Build history of the part. All positions in model axes, mm. A direction names the side the tool comes from. Give positions to 0.01 mm unless a question says otherwise; leave off trailing zeros. Loops run counter-clockwise (first coordinate to the right, second up) from the corner with the lowest first, then second, coordinate; pieces in that order, holes last. Notation, with made-up numbers: (-20.5, 85) -> (7.5, 85) arc R26 cw to (7.5, 112) -> close; hole circle Ø4 at (51, 73). An arc over 180 degrees is marked (long way). One line per question, with ' | ' between items. Start each with the question number.
(1) Flat gauge pin, fed straight in: pin 1 Ø3 at (x, y) = (50, 15.5) entering from -Z. Where does the tip first touch, or does it go through?
(2) Slice it at A-A, the plane x = 50. Write the cut outline in (y, z).
(3) Drill centre lines: L1, parallel to X at y = 15, z = 8.25; L2, parallel to Y at x = 50, z = 91. Where is each one in solid material? Low to high. Write a range as from..to.
(4) 3-axis set-ups, long thin cutter, end or side, ignore diameter. For faces 4 (the face through (47.6, 16.8, 5.9)), 5 (the face through (49, 0, 49)), 6 (the face through (50, 15, 88)): which of +Z, -Z, +X, -X, +Y, -Y reach the whole face in a straight line?
(5) Mould opens along X. For faces 1 (the face through (50, 15, 12)), 2 (the face through (49, 30, 49)), 3 (the face through (100, 15, 49)) say: pulls with the +X half, pulls with the -X half, needs draft (parallel to the pull), parting line crosses it, or undercut.
```python
from build123d import *

# Parameters (mm, degrees)
F0_W     = 100
F0_H     = 30
F1_DEPTH = 100
F2_R     = 3
F3_DEPTH = 12
F4_R     = 3
F5_DEPTH = 12


with BuildPart() as f1:
    # F0 (on Top) → F1 (new body)
    with BuildSketch(Plane.XY):
        with Locations((50, 15)):
            Rectangle(F0_W, F0_H)
    extrude(amount=F1_DEPTH)

    # F2 (on face) → F3 (cut)
    with BuildSketch(Plane(origin=(0, 0, 0), x_dir=(1, 0, 0), z_dir=(0, 0, -1))):
        with Locations((50, -15)):
            Circle(F2_R)
    extrude(amount=-F3_DEPTH, mode=Mode.SUBTRACT)

    # F4 (on face) → F5 (cut)
    with BuildSketch(Plane.XY.offset(100)):
        with Locations((50, 15)):
            Circle(F4_R)
    extrude(amount=-F5_DEPTH, mode=Mode.SUBTRACT)


solid = f1.part
```
Final values:
1) pin 1: z = 12
2) outline: (0, 0) -> (12, 0) -> (12, 12) -> (18, 12) -> (18, 0) -> (30, 0) -> (30, 100) -> (18, 100) -> (18, 88) -> (12, 88) -> (12, 100) -> (0, 100) -> close
3) L1: 0..47, 53..100 | L2: 0..12, 18..30
4) face 4: -Z | face 5: +Z, -Z, +X, -X, -Y | face 6: +Z
5) face 1: undercut | face 2: needs draft | face 3: pulls with the +X half
